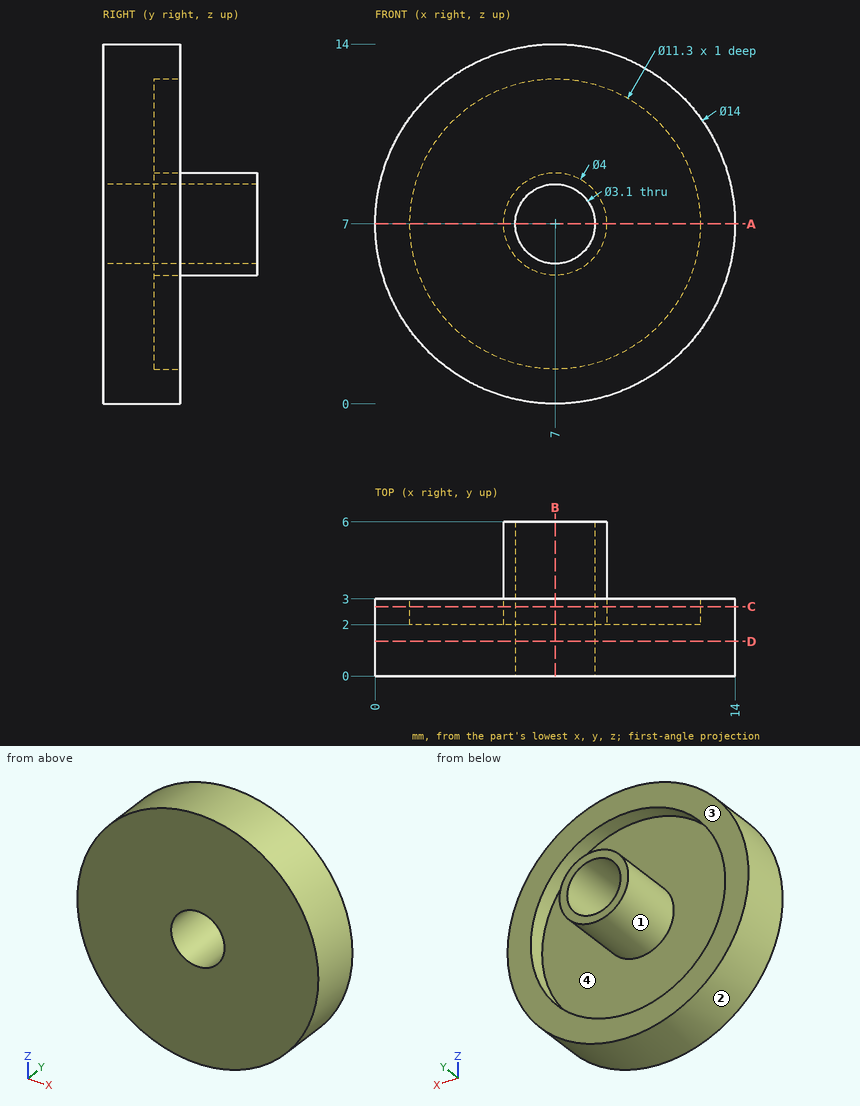
Drawing for the job (mm, zero at the part's lowest x, y, z). Round coordinates to 2 decimals unless told otherwise and drop trailing zeros. Write each loop counter-clockwise with the first axis right and the second up, starting at its lowest first coordinate (ties: lowest second). Pieces come first, ordered by that corner, then holes. Notation, with made-up numbers: M 50,23.5 L 80,23.5 A10 cw 80,42.5 Z; hole C 9,-37.5 d10. An arc over 180 degrees is marked long. Put each result on its own line as item: value.
Item 1: Mould opens along X. For the marked faces 1, 2, 3 and 4 say: +X half, -X half, draft (parallel to the pull), parting line (faces both ways), or undercut.
Responses:
face 1: undercut
face 2: parting line
face 3: draft
face 4: undercut
Item 2: Cut at A-A (z = 7). List the corners of the cut face in (x, y).
Responses:
outline: M 0,0 L 5.45,0 L 5.45,6 L 5,6 L 5,2 L 1.35,2 L 1.35,3 L 0,3 Z; M 8.55,0 L 14,0 L 14,3 L 12.65,3 L 12.65,2 L 9,2 L 9,6 L 8.55,6 Z
Item 3: Probe L1, parallel to X at y = 2.6, z = 7; L2, parallel to Z at x = 7, y = 1.9. List the from-to ranges inside material, lowest first. Write a range as from..to.
Responses:
L1: 0..1.35, 5..5.45, 8.55..9, 12.65..14
L2: 0..5.45, 8.55..14
Item 4: Cut at B-B (x = 7). List the corners of the cut face in (y, z), and give its area (3 significant figures).
Responses:
outline: M 0,0 L 3,0 L 3,1.35 L 2,1.35 L 2,5 L 6,5 L 6,5.45 L 0,5.45 Z; M 0,8.55 L 6,8.55 L 6,9 L 2,9 L 2,12.65 L 3,12.65 L 3,14 L 0,14 Z
area: 28.1 mm²
Item 5: Cut at C-C (y = 2.7). List the corners of the cut face in (x, z).
Responses:
outline: C 7,7 d14; C 7,7 d4; hole C 7,7 d11.3; hole C 7,7 d3.1
Item 6: Flat gauge pins, fed straight in: P1, Ø1, axis at y = 4, z = 2.5, coming from the -X side; P2, Ø4, axis at x = 1.5, z = 11.5, coming from the -Y side; P3, Ø1.5, axis at y = 1.5, z = 12, coming from the +X side; P4, Ø6, axis at x = 9, z = 12, coming from the +Y side. Where does each tip first touch, or does it go through?
Responses:
P1: through
P2: y = 0
P3: x = 12.56
P4: y = 3
Item 7: Cut at D-D (y = 1.35). List the corners of the cut face in (x, z).
Responses:
outline: C 7,7 d14; hole C 7,7 d3.1
